Part model, mm, in its own coordinate system. A direction names the side the tool comes from. Coordinates: 2 decimals unless noted, no trailing zeros. Loops run counter-clockwise (first coordinate to the right, second up) from the corner with the lowest first, then second, coordinate; pieces in that order, holes last. Notation, with made-up numbers: M -30.75,-30 L 20.25,-30 A24 cw 20.25,-10 Z; hole C 57,-19 d1. An arc over 180 degrees is marked long. Use CSV: the item, a comma, the result in double quotes. Start each with the question number.
from build123d import *

# Parameters (mm, degrees)
SKETCH1_R           = 14.2875
SKETCH1_R_2         = 4.7625
BOSS_EXTRUDE1_DEPTH = 7.9248
SKETCH2_R           = 15.875
SKETCH2_R_2         = 14.2875
BOSS_EXTRUDE2_DEPTH = 1.5748
CHAMFER1_SIZE       = 1.27


with BuildPart() as part:
    # Sketch1 → Boss-Extrude1 (new body)
    with BuildSketch(Plane(origin=(0, 0, 0), x_dir=(1, 0, 0), z_dir=(0, 1, 0))):
        Circle(SKETCH1_R)
        Circle(SKETCH1_R_2, mode=Mode.SUBTRACT)
    extrude(amount=BOSS_EXTRUDE1_DEPTH)

    # Sketch2 → Boss-Extrude2 (add)
    with BuildSketch(Plane.XZ):
        Circle(SKETCH2_R)
        Circle(SKETCH2_R_2, mode=Mode.SUBTRACT)
    extrude(amount=-BOSS_EXTRUDE2_DEPTH)

    # Chamfer1
    chamfer1_edges = [part.edges().sort_by_distance(p)[0] for p in [
        (-14.2875, 7.9248, 0),
    ]]
    chamfer(chamfer1_edges, length=CHAMFER1_SIZE)


solid = part.part
1. Pin check, flat tip, straight feed: pin 1 (2 mm diameter, centred on x = -3, y = 3.5, fed in from -Z). Stop position of the tip, or through.
2. Slice it at A-A, the plane x = 0. List the corners of the cut face in (y, z) (1 decimal), and give its area (3 significant figures).
3. Wall check: probe 1 along Z at (x, y) = (0, 6); probe 2 along Z at (x, y) = (0, 1.5) (1 decimal). Give the ranges that are in metal, low to high.
4. Slice it at C-C, the plane y = 4.75. List the corners of the cut face in (x, z) (1 decimal), and give its area (3 significant figures).
5. Tool access for faces 1 (the face through (6, 7.925, 0)), 2 (the face through (-11.83, 1.575, 8.31)): list every direction of +Z, -Z, +X, -X, +Y, -Y with a clear straight run to the whole face (end or side of a thin tool).
6. Two-plate mould, pull along Z, no slides. Class faces 3 (the face through (-3.78, 3.91, 2.9)), 4 (the face through (-3.441, 0.776, -15.497)), 5 (the face through (3, 0, 4)): pulls with the +Z half, pulls with the -Z half, needs draft (parallel to the pull), parting line crosses it, or undercut.
7. Slice it at B-B, the plane z = 0. List the corners of the cut face in (x, y) (1 decimal), and give its area (3 significant figures).
Found:
1,pin 1,"z = -14.15"
2,outline,"M 0,-15.9 L 1.6,-15.9 L 1.6,-14.3 L 6.7,-14.3 L 7.9,-13 L 7.9,-4.8 L 0,-4.8 Z; M 0,4.8 L 7.9,4.8 L 7.9,13 L 6.7,14.3 L 1.6,14.3 L 1.6,15.9 L 0,15.9 Z"
2,area,"154 mm^2"
3,probe 1,"-14.29 to -4.76, 4.76 to 14.29"
3,probe 2,"-15.9 to -4.8, 4.8 to 15.9"
4,outline,"C 0,0 d28.6; hole C 0,0 d9.5"
4,area,"570 mm^2"
5,face 1,"+Z, -Z, +X, -X, +Y"
5,face 2,"+Y"
6,face 3,"undercut"
6,face 4,"parting line crosses it"
6,face 5,"needs draft"
7,outline,"M -15.9,0 L -4.8,0 L -4.8,7.9 L -13,7.9 L -14.3,6.7 L -14.3,1.6 L -15.9,1.6 Z; M 4.8,0 L 15.9,0 L 15.9,1.6 L 14.3,1.6 L 14.3,6.7 L 13,7.9 L 4.8,7.9 Z"
7,area,"154 mm^2"
